The listing builds one solid part. Answer for the finished solid, in the listing's coordinates (mm). Face numbers are marked on the shaded views. A direction names the side the tool comes from. Round coordinates to 2 decimals unless told otherwise and drop trailing zeros. Write each loop counter-clockwise with the first axis right and the second up, starting at its lowest first coordinate (ties: lowest second). Pieces come first, ordered by that corner, then holes.
Item 1: Find section D-D on y = 16.75. Give the number of separate pieces and of enclosed holes in the cut face, then the cut area to 3 significant figures.
Item 2: Find section A-A on z = 9.75. Give the vertices of the cut face in (x, y) (3 decimals), then the cut area to 3 significant figures.
Item 3: Find the intervals of material crossed by probe 1 along X at (y, z) = (11, 2); probe 2 along Y at (x, z) = (-20, -12) (3 decimals); probe 3 along Z at (x, y) = (-3.5, 8.5), in increasing order.
Item 4: Each of these flat-tipped pins is pushed along its axis until it touches: pin 1 (6.5 mm diameter, centred on x = -20.53, z = 0, fed in from -Y) (3 decimals); pin 2 (12 mm diameter, centred on x = -7.5, z = -2, fed in from +Y) (3 decimals); pin 3 (5 mm diameter, centred on x = -20.53, z = 0, fed in from +Y); pin 4 (4 mm diameter, centred on y = 4, z = 5, fed in from -X). Where does it stop, or does it pass through?
Item 5: Find section B-B on x = -18. Give the vertices of the cut face in (y, z) (3 decimals), then the cut area to 3 significant figures.
Item 6: For a pull along Y with two mould halves and no side action, classify the marked faces 1, 2 and 3 as +Y half, -Y half, draft (parallel to the pull), parting line (faces both ways), or undercut.
Item 7: A tool of negligible diameter and unlimited length cuts with its end or side. For the marked faces 4, 5 and 6, from which of +Z, -Z, +X, -X, +Y, -Y can it reach the whole face along a straight path? Write none if from no direction.
Item 8: Find section C-C on y = 6. Give the vertices of the cut face in (x, z).
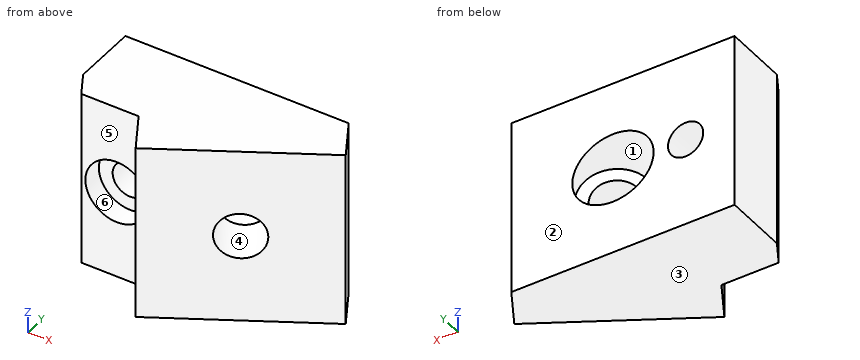
```python
from build123d import *

# Parameters (mm, degrees)
ESBO_O1_W                  = 30
ESBO_O1_H                  = 30
RESSALTO_EXTRUS_O1_DEPTH   = 22.775
CORTE_EXTRUS_O1_DEPTH      = 41.542577927
ESBO_O3_OUTSIDE_W          = 48.998
ESBO_O3_OUTSIDE_H          = 41.63
ESBO_O3_OUTSIDE_W_2        = 30
ESBO_O3_OUTSIDE_H_2        = 30
CORTE_EXTRUS_O2_DEPTH      = 30.010251575
RESSALTO_EXTRUS_O2_DEPTH   = 30
ESBO_O5_R                  = 3.95
CORTE_EXTRUS_O3_DEPTH      = 32.012511133
CORTE_EXTRUS_O5_START      = -8
ESBO_O8_R                  = 6
CORTE_EXTRUS_O5_DEPTH      = 25
ESBO_O9_R                  = 3.95
CORTE_EXTRUS_O6_DEPTH      = 10
RESSALTO_EXTRUS_O3_DEPTH   = 15
ESBO_O11_W                 = 30
ESBO_O11_H                 = 15
RESSALTO_EXTRUS_O4_DEPTH   = 10
ESBO_O9_2_R                = 3.95
CORTE_EXTRUS_O7_DEPTH      = 30
ESBO_O12_R                 = 5.35
CORTE_EXTRUS_O8_DEPTH      = 10
CORTE_EXTRUS_O8_DEPTH_BACK = 3.5
ESBO_O13_W                 = 11.908257902
ESBO_O13_H                 = 30
CORTE_EXTRUS_O9_DEPTH      = 23.5
ESBO_O14_R                 = 3.95
ESBO_O14_R_2               = 3
RESSALTO_EXTRUS_O5_DEPTH   = 11.5
CORTE_EXTRUS_O10_DEPTH     = 30


with BuildPart() as part:
    # Esbo_o1 → Ressalto-extrus_o1 (new body)
    with BuildSketch(Plane(origin=(0, 0, 0), x_dir=(1, 0, 0), z_dir=(0, 1, 0))):
        Rectangle(ESBO_O1_W, ESBO_O1_H)
    extrude(amount=RESSALTO_EXTRUS_O1_DEPTH)

    # Esbo_o2 → Corte-extrus_o1 (cut, through all)
    with BuildSketch(Plane.XY.offset(15)):
        Polygon((-15, 0), (15, 17.320508076), (15, 0), align=None)
    extrude(amount=-CORTE_EXTRUS_O1_DEPTH, mode=Mode.SUBTRACT)

    # Esbo_o3 outside → Corte-extrus_o2 (cut, through all)
    with BuildSketch(Plane(origin=(-3.75, 6.495190528, 0), x_dir=(0.8660254037844378, 0.5000000000000017, 0), z_dir=(0.5000000000000016, -0.8660254037844377, 0))):
        with Locations((5.694, 0)):
            Rectangle(ESBO_O3_OUTSIDE_W, ESBO_O3_OUTSIDE_H)
        with Locations((4.330127019, 0)):
            Rectangle(ESBO_O3_OUTSIDE_W_2, ESBO_O3_OUTSIDE_H_2, mode=Mode.SUBTRACT)
    extrude(amount=-CORTE_EXTRUS_O2_DEPTH, mode=Mode.SUBTRACT)

    # Esbo_o4 → Ressalto-extrus_o2 (add)
    with BuildSketch(Plane.XY.offset(15)):
        Polygon((-25.469660456, 22.775), (-15, 4.641016151), (-15, 22.775), align=None)
    extrude(amount=-RESSALTO_EXTRUS_O2_DEPTH)

    # Esbo_o5 → Corte-extrus_o3 (cut, through all)
    with BuildSketch(Plane(origin=(-3.75, 6.495190528, 0), x_dir=(-0.8660254037844379, -0.5000000000000013, 0), z_dir=(0.5000000000000013, -0.8660254037844379, 0))):
        with Locations(Location((-4.330131096, -4.077e-06, 0), (0, 0, 180))):
            Circle(ESBO_O5_R)
    extrude(amount=-CORTE_EXTRUS_O3_DEPTH, mode=Mode.SUBTRACT)

    # Esbo_o8 → Corte-extrus_o5 (cut)
    with BuildSketch(Plane(origin=(-3.75, 6.495190528, 0), x_dir=(0.8660254037844379, 0.5000000000000013, 0), z_dir=(0.5000000000000013, -0.8660254037844379, 0)).offset(CORTE_EXTRUS_O5_START)):
        with Locations((4.330131096, 4.077e-06)):
            Circle(ESBO_O8_R)
    extrude(amount=-CORTE_EXTRUS_O5_DEPTH, mode=Mode.SUBTRACT)

    # Esbo_o9 → Corte-extrus_o6 (cut)
    with BuildSketch(Plane(origin=(0, 22.775, 0), x_dir=(1, 0, 0), z_dir=(0, 1, 0))):
        with Locations(Location((-20.527350903, 0, 0), (0, 0, 270))):
            Circle(ESBO_O9_R)
    extrude(amount=-CORTE_EXTRUS_O6_DEPTH, mode=Mode.SUBTRACT)



with BuildPart() as body_2:
    # Esbo_o10 → Ressalto-extrus_o3 (new body)
    with BuildSketch(Plane(origin=(0, 22.775, 0), x_dir=(1, 0, 0), z_dir=(0, 1, 0))):
        Polygon((-25.469660456, 15), (-40.785608805, 15), (-40.785608805, -15), (-25.469660456, -15), (-25.469660456, -3.937347933), (-25.469660456, 3.937339779), align=None)
    extrude(amount=-RESSALTO_EXTRUS_O3_DEPTH)


with BuildPart() as part_1:
    add(part.part)

    add(body_2.part)  # Ressalto-extrus_o4 merges body 2
    # Esbo_o11 → Ressalto-extrus_o4 (add)
    with BuildSketch(Plane(origin=(-25.469660456, 0, 0), x_dir=(0, 0, -1), z_dir=(1, 0, 0))):
        with Locations((0, 15.275)):
            Rectangle(ESBO_O11_W, ESBO_O11_H)
    extrude(amount=RESSALTO_EXTRUS_O4_DEPTH)

    # Esbo_o9_2 → Corte-extrus_o7 (cut)
    with BuildSketch(Plane(origin=(0, 22.775, 0), x_dir=(1, 0, 0), z_dir=(0, 1, 0))):
        with Locations(Location((-20.527350903, 0, 0), (0, 0, 270))):
            Circle(ESBO_O9_2_R)
    extrude(amount=-CORTE_EXTRUS_O7_DEPTH, mode=Mode.SUBTRACT)

    # Esbo_o12 → Corte-extrus_o8 (cut, two sides)
    with BuildSketch(Plane.XZ.offset(-7.775)) as corte_extrus_o8_sk:
        with Locations(Location((-20.527350903, 0, 0), (0, 0, 45.977333205))):
            Circle(ESBO_O12_R)
    extrude(amount=CORTE_EXTRUS_O8_DEPTH, mode=Mode.SUBTRACT)
    extrude(corte_extrus_o8_sk.sketch, amount=-CORTE_EXTRUS_O8_DEPTH_BACK, mode=Mode.SUBTRACT)

    # Esbo_o13 → Corte-extrus_o9 (cut)
    with BuildSketch(Plane.XZ.offset(-7.775)):
        with Locations((-34.831479854, 0)):
            Rectangle(ESBO_O13_W, ESBO_O13_H)
    extrude(amount=-CORTE_EXTRUS_O9_DEPTH, mode=Mode.SUBTRACT)

    # Esbo_o14 → Ressalto-extrus_o5 (add)
    with BuildSketch(Plane.XZ.offset(-11.275)):
        with Locations((-20.527350903, 0)):
            Circle(ESBO_O14_R)
        with Locations(Location((-20.527350903, 0, 0), (0, 0, 270))):
            Circle(ESBO_O14_R_2, mode=Mode.SUBTRACT)
    extrude(amount=-RESSALTO_EXTRUS_O5_DEPTH)

    # Esbo_o15 → Corte-extrus_o10 (cut)
    with BuildSketch(Plane.XY.offset(15)):
        Polygon((-38.655450544, 28.698110147), (-22.922361913, 1.447601278), (-38.655450544, 1.447601278), align=None)
    extrude(amount=-CORTE_EXTRUS_O10_DEPTH, mode=Mode.SUBTRACT)


solid = part_1.part
```
Check values:
1. separate pieces: 1
1. enclosed holes: 2
1. area: 1,110 mm2
2. outline: (-28.877, 11.762) - (-26.575, 7.775) - (-16.809, 7.775) - (-12.99, 1.16) - (12.99, 16.16) - (9.171, 22.775) - (-28.877, 22.775) - close
2. area: 600 mm2
3. probe 1: x = -28.44 to -25.49, -15.57 to -5.28, 2.58 to 4.05
3. probe 2: y = 7.775 to 22.775
3. probe 3: z = -15 to -2.43, 2.43 to 15
4. pin 1: stops at y = 11.275
4. pin 2: stops at y = 22.775
4. pin 3: passes through
4. pin 4: stops at x = -15.78
5. outline: (7.775, -15) - (22.775, -15) - (22.775, -1.616) - (11.275, -1.616) - (11.275, -4.715) - (7.775, -4.715) - close; (7.775, 4.715) - (11.275, 4.715) - (11.275, 1.616) - (22.775, 1.616) - (22.775, 15) - (7.775, 15) - close
5. area: 380 mm2
6. face 1: undercut
6. face 2: +Y half
6. face 3: draft
7. face 4: none
7. face 5: +Z, -Z, -X, -Y
7. face 6: -Y
8. outline: (-15.78, -15) - (-4.61, -15) - (-4.61, 15) - (-15.78, 15) - (-15.78, 2.48) arc R5.35 cw to (-15.78, -2.48) - close
